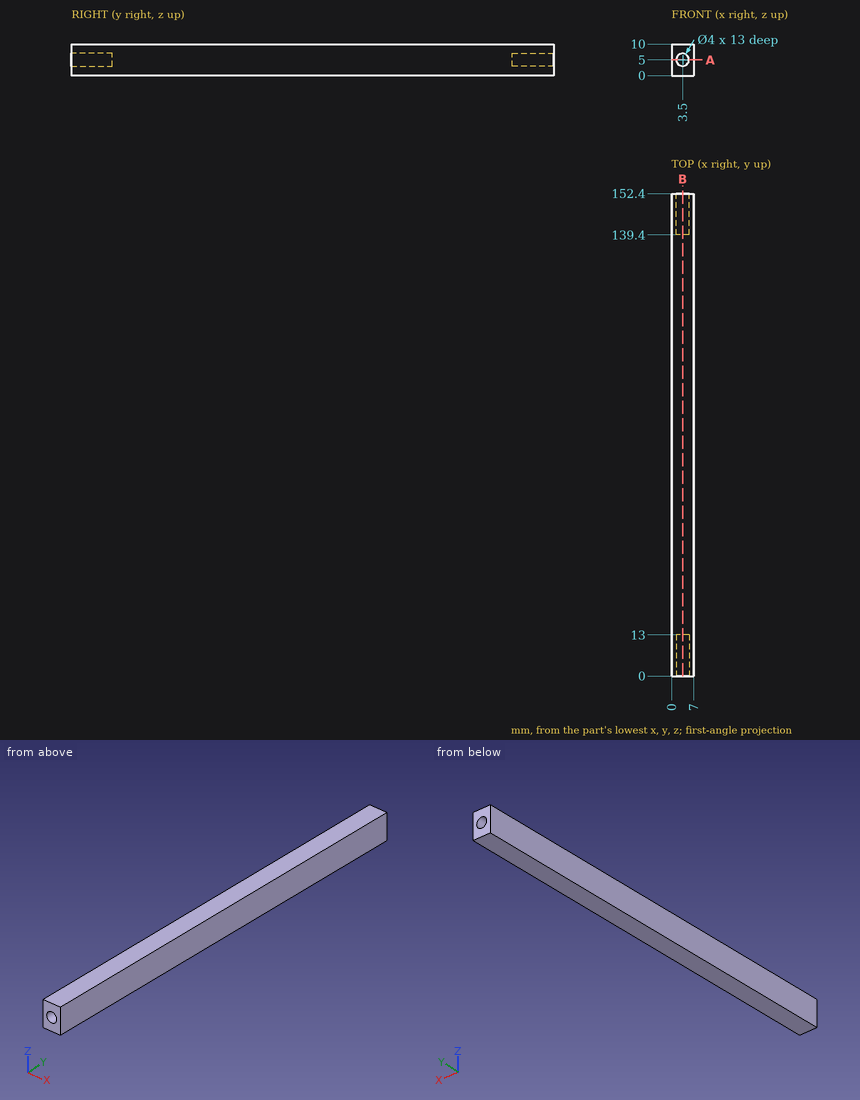
The figure shows three views and two pictorial views of one solid part (mm, origin at its lowest corner). Answer the questions. Coordinates: 2 decimals unless noted, no trailing zeros. Loops run counter-clockwise (first coordinate to the right, second up) from the corner with the lowest first, then second, coordinate; pieces in that order, holes last.
1) Flat-ended cylindrical pins translate along their axes: pin 1 Ø2 at (x, z) = (3, 5) entering from -Y; pin 2 Ø2 at (x, z) = (3, 5) entering from +Y. Find the tip coordinate at first contact, or state that the pin passes through.
2) Find section A-A on z = 5. Write down the section's boundary in (x, y), then the cut area to 3 significant figures.
3) Find section B-B on x = 3.5. Write down the section's boundary in (y, z), then the cut area to 3 significant figures.
4) Find the intervals of material crossed by L1, parallel to X at y = 145.5, z = 5; L2, parallel to X at y = 144.5, z = 6.5; L3, parallel to Y at x = 3.75, z = 6.25, in increasing order.
Values:
1. pin 1: stops at y = 13
1. pin 2: stops at y = 139.4
2. outline: (0, 0) - (1.5, 0) - (1.5, 13) - (5.5, 13) - (5.5, 0) - (7, 0) - (7, 152.4) - (5.5, 152.4) - (5.5, 139.4) - (1.5, 139.4) - (1.5, 152.4) - (0, 152.4) - close
2. area: 963 mm2
3. outline: (0, 0) - (152.4, 0) - (152.4, 3) - (139.4, 3) - (139.4, 7) - (152.4, 7) - (152.4, 10) - (0, 10) - (0, 7) - (13, 7) - (13, 3) - (0, 3) - close
3. area: 1,420 mm2
4. L1: x = 0 to 1.5, 5.5 to 7
4. L2: x = 0 to 2.18, 4.82 to 7
4. L3: y = 13 to 139.4
